Geometry check sheet. Reference: the model listing, model coordinates, mm. Round coordinates to 2 decimals unless told otherwise and drop trailing zeros. Loops run counter-clockwise (first coordinate to the right, second up) from the corner with the lowest first, then second, coordinate; pieces in that order, holes last. Notation, with made-up numbers: (3.25, 10.25) - (40.25, 10.25) arc R25 ccw to (40.25, 36.25) - close; hole circle Ø10 at (-18.75, -14.75). An arc over 180 degrees is marked (long way). Answer as CSV lines item,"result". Start each with the question number.
1) Cross-section at C-C on x = 55. Record the boundary of the cut face in (y, z), and give its area (3 significant figures).
2) Cross-section at A-A on y = 17.5. Record the boundary of the cut face in (x, z).
3) Cross-section at B-B on z = 70.5. Record the boundary of the cut face in (x, y), and give its area (3 significant figures).
4) Depth check by flat-ended pin: P1, Ø3, axis at y = 52.5, z = 29.5, coming from the +X side. Enter the tip coordinate at first touch or a pass-through.
5) Thickness scan on line 1 along X through (y, z) = (28, 76); line 2 along X through (y, z) = (59, 37.5); line 3 along Y through (x, z) = (58, 30.5). Record the ranges inside material, lowest first.
6) Cross-section at D-D on y = 7. Record the boundary of the cut face in (x, z).
from build123d import *

# Parameters (mm, degrees)
F1_DEPTH = 88


with BuildPart() as f1:
    # F0 (on Top) → F1 (new body)
    with BuildSketch(Plane.XY):
        with BuildLine():
            Line((0, 75), (0, 0))
            Line((0, 0), (50, 0))
            ThreePointArc((50, 0), (87.5, 37.5), (50, 75))
            Line((50, 75), (0, 75))
        make_face()
        with BuildLine():
            ThreePointArc((75, 37.5), (67.67767, 19.82233), (50, 12.5))
            ThreePointArc((50, 12.5), (25, 37.5), (50, 62.5))
            ThreePointArc((50, 62.5), (67.67767, 55.17767), (75, 37.5))
        make_face(mode=Mode.SUBTRACT)
    extrude(amount=F1_DEPTH)


solid = f1.part
Answer block:
1,outline,"(0.33, 0) - (13.01, 0) - (13.01, 88) - (0.33, 88) - close; (61.99, 0) - (74.67, 0) - (74.67, 88) - (61.99, 88) - close"
1,area,"2,230 mm^2"
2,outline,"(0, 0) - (35, 0) - (35, 88) - (0, 88) - close; (65, 0) - (81.72, 0) - (81.72, 88) - (65, 88) - close"
3,outline,"(0, 0) - (50, 0) arc R37.5 ccw to (50, 75) - (0, 75) - close; hole (50, 12.5) arc R25 ccw to (75, 37.5) arc R25 ccw to (50, 62.5) arc R25 ccw to start"
3,area,"4,000 mm^2"
4,P1,"stops at x = 84.99"
5,line 1,"x = 0 to 26.88, 73.12 to 86.28"
5,line 2,"x = 0 to 37.24, 62.76 to 80.72"
5,line 3,"y = 0.86 to 13.81, 61.19 to 74.14"
6,outline,"(0, 0) - (71.82, 0) - (71.82, 88) - (0, 88) - close"
